Autodesk Inventor part; units mm, degrees
ref_plane "YZ Plane" through (0, 0, 0) normal (1, 0, 0) x (0, 1, 0)
ref_plane "XZ Plane" through (0, 0, 0) normal (0, 1, 0) x (-1, 0, 0)
ref_plane "XY Plane" through (0, 0, 0) normal (0, 0, 1) x (1, 0, 0)
sketch "Sketch1" plane through (0, 0, 0) normal (0, 0, 1) x (1, 0, 0)
  line L0 (0, 0) -> (0, 200) construction
  arc A0 (37.1934, 204.7857) -> (-37.1934, 204.7857) centre (0, 200) ccw
  line L1 (0, 200) -> (-18.25, 200) construction
  circle A1 centre (-18.25, 200) radius 2.5
  line L2 (0, 200) -> (18.25, 200) construction
  circle A2 centre (18.25, 200) radius 2.5
  circle A3 centre (0, 0) radius 15 construction
  line L3 (37.1934, 204.7857) -> (59.7122, 29.7756)
  line L4 (-37.1934, 204.7857) -> (-59.9286, 28.0941)
  line L5 (48.4528, 117.2807) -> (43.4937, 116.6426) construction
  line L6 (51.1509, 57.1332) -> (35.8365, 176.152) construction
  circle A4 centre (35.8365, 176.152) radius 1.5
  circle A5 centre (51.1509, 57.1332) radius 1.5
  circle A6 centre (43.4937, 116.6426) radius 1.5
  line L7 (0, 237.5) -> (0, 232.5) construction
  circle A7 centre (0, 232.5) radius 1.5
  circle A8 centre (-35.8365, 176.152) radius 1.5
  circle A9 centre (-43.4937, 116.6426) radius 1.5
  circle A10 centre (-51.1509, 57.1332) radius 1.5
  circle A11 centre (0, 200) radius 4.75
  circle A12 centre (0, 0) radius 45 construction
  circle A13 centre (0, -45) radius 9.5
  circle A14 centre (0, -45) radius 14.5 construction
  circle A15 centre (0, -59.5) radius 2.25 construction
  circle A16 centre (14.5, -45) radius 2.25 construction
  circle A17 centre (0, -30.5) radius 2.25 construction
  circle A18 centre (-14.5, -45) radius 2.25 construction
  circle A19 centre (0, -45) radius 21.5 construction
  circle A20 centre (38.9711, 22.5) radius 21.5 construction
  circle A21 centre (51.5285, 29.75) radius 2.25 construction
  circle A22 centre (46.2211, 9.9426) radius 2.25 construction
  circle A23 centre (31.7211, 35.0574) radius 2.25 construction
  circle A24 centre (26.4138, 15.25) radius 2.25 construction
  circle A25 centre (38.9711, 22.5) radius 9.5
  circle A26 centre (-38.9711, 22.5) radius 21.5 construction
  circle A27 centre (-51.5285, 29.75) radius 2.25 construction
  circle A28 centre (-31.7211, 35.0574) radius 2.25 construction
  circle A29 centre (-46.2211, 9.9426) radius 2.25 construction
  circle A30 centre (-26.4138, 15.25) radius 2.25 construction
  circle A31 centre (-38.9711, 22.5) radius 9.5
  line L8 (-18.6195, -55.75) -> (-57.5907, 11.75)
  line L9 (18.6195, -55.75) -> (57.5907, 11.75)
  line L10 (48.4528, 117.2807) -> (48.4528, 23.0901) construction
  line L11 (59.7122, 29.7756) -> (60.2953, 25.2438)
  line L12 (48.4528, 23.0901) -> (48.4528, -26.9099) construction
  line L13 (48.4528, -26.9099) -> (38.566, -21.2018) construction
  line L14 (38.566, -21.2018) -> (34.2359, -18.7018) construction
  circle A32 centre (34.2359, -18.7018) radius 1.5
  circle A33 centre (-34.2359, -18.7018) radius 1.5
  arc A34 (57.5907, 11.75) -> (60.2953, 25.2438) centre (38.9711, 22.5) ccw
  arc A35 (-60.2953, 25.2438) -> (-57.5907, 11.75) centre (-38.9711, 22.5) ccw
  arc A36 (-18.6195, -55.75) -> (18.6195, -55.75) centre (0, -45) ccw
  line L15 (38.9711, 22.5) -> (53.4711, 22.5) construction
  line L16 (-59.9286, 28.0941) -> (-60.2953, 25.2438)
  circle A37 centre (0, 0) radius 5.1
  line L17 (0, 0) -> (0, -8) construction
  circle A38 centre (0, -8) radius 1.75
  circle A39 centre (8, 0) radius 1.75
  circle A40 centre (0, 8) radius 1.75
  circle A41 centre (-8, 0) radius 1.75
  line L18 (0, 200) -> (0, 135) construction
  circle A42 centre (-27, 96) radius 1.1
  circle A43 centre (-23.9586, 105) radius 1.1
  dimension "d84" = 90
  dimension "d86" = 29
  dimension "d58" = 200
  dimension "d59" = 75
  dimension "d60" = 18.25
  dimension "d61" = 5
  dimension "d62" = 30
  dimension "d63" = 5
  dimension "d64" = 120
  dimension "d65" = 3
  dimension "d66" = 3
  dimension "d67" = 3
  dimension "d68" = 5
  dimension "d69" = 3
  dimension "d70" = 9.5
  dimension "d85" = 19
  dimension "d87" = 4.5
  dimension "d88" = 45
  dimension "d89" = 14.5
  dimension "d90" = 14.5
  dimension "d91" = 360
  dimension "d92" = 43
  dimension "d93" = 360
  dimension "d94" = 94.1906
  dimension "d95" = 50
  dimension "d96" = 5
  dimension "d97" = 3
  dimension "d103" = 10.2
  dimension "d104" = 8
  dimension "d105" = 3.5
  dimension "d108" = 360
  dimension "d110" = 65
  dimension "d113" = 2.2
  dimension "d115" = 2.2
  dimension "d116" = 27
  dimension "d118" = 9.5
  dimension "d119" = 95
  dimension "d120" = 104
extrude "Extrusion1" add sketch "Sketch1" along normal blind 4
sketch "Sketch2" plane through (0, 0, 4) normal (0, 0, 1) x (1, 0, 0)
  line L0 (0, 0) -> (0, -60) construction
  line L1 (0.05, -59.95) -> (-0.05, -59.95)
  line L2 (-0.05, -59.95) -> (-0.05, -60.05)
  line L3 (-0.05, -60.05) -> (0.05, -60.05)
  line L4 (0.05, -60.05) -> (0.05, -59.95)
  line L5 (0.05, -59.95) -> (-0.05, -60.05) construction
  line L6 (-0.05, -59.95) -> (0.05, -60.05) construction
  dimension "d47" = 60
  dimension "d48" = 0.1
  dimension "d49" = 0.1
extrude "Extrusion2" add sketch "Sketch2" along normal blind 0.1
equation "\"d63\" = d101"
equation "\"d65\" = d102"
equation "\"d66\" = d102"
equation "\"d67\" = d102"
equation "\"d68\" = d101"
equation "\"d69\" = d102"
equation "\"d96\" = d101"
equation "\"d97\" = d102"
properties part number "2ELO"
Input: part model. Units: mm. Frame: model coordinates. Coordinates: 2 decimals unless noted, no trailing zeros. Write each loop counter-clockwise with the first axis right and the second up, starting at its lowest first coordinate (ties: lowest second). Pieces come first, ordered by that corner, then holes. Notation, with made-up numbers: (75.5, 65) - (86.5, 65) arc R29 cw to (86.5, 95) - close; hole circle Ø9 at (31, 62.5). An arc over 180 degrees is marked (long way). Put each result on its own line as item: value. Start each with the question number.
1) Ray query, L1, parallel to X at y = 22, z = 0.5; L2, parallel to X at y = 29, z = 3.55; L3, parallel to Y at x = 8, z = 2.8. Return the intervals inside material, ascending.
2) Cut plane C-C (y = 89.5). Return the cut outline in (x, z), plus the area to 3 significant figures.
3) Contact query for flat-ended pins moving along their axis: pin 1 (3 mm diameter, centred on x = 26, y = 54, fed in from +Z); pin 2 (2 mm diameter, centred on x = -19.5, z = 2.5, fed in from +Y). Output: stop coordinate, or through.
4) Cut plane B-B (x = 25.5). Return the cut outline in (y, z), plus the area to 3 significant figures.
5) Cut plane A-A (z = 3.3). State how many separate pieces and enclosed holes the cut face has, plus the area to 3 significant figures.
Resolved:
1. L1: x = -60.47 to -48.46, -29.48 to 29.48, 48.46 to 60.47
1. L2: x = -59.81 to -45.9, -32.04 to 32.04, 45.9 to 59.81
1. L3: y = -64.96 to -50.12, -39.88 to -1.75, 1.75 to 236.64
2. outline: (-52.03, 0) - (52.03, 0) - (52.03, 4) - (-52.03, 4) - close
2. area: 416 mm2
3. pin 1: stops at z = 4
3. pin 2: stops at y = 232.62
4. outline: (-43.83, 0) - (227.5, 0) - (227.5, 4) - (-43.83, 4) - close
4. area: 1,090 mm2
5. separate pieces: 1
5. enclosed holes: 22
5. area: 25,200 mm2
